from build123d import *

# Parameters (mm, degrees)
ESBO_O6_R                 = 10.25
ESBO_O6_R_2               = 8.55
FURO_ROSCADO_DE_M61_D     = 5
FURO_ROSCADO_DE_M61_DEPTH = 15
FURO_ROSCADO_DE_M61_TIP   = 1.502151548


with BuildPart() as part:
    # Varredura1: sweep along a path in Esboço5
    with BuildLine(Plane.XY) as varredura1_path:
        Line((0, 0), (-160, 0))
        ThreePointArc((-160, 0), (-174.142135624, 5.857864376), (-180, 20))
        Line((-180, 20), (-180, 260))
    # Esboço6 → Varredura1 (sweep)
    with BuildSketch(Plane.ZY):
        Circle(ESBO_O6_R)
        Circle(ESBO_O6_R_2, mode=Mode.SUBTRACT)
    sweep(path=varredura1_path.line)

    # Furo roscado de M61
    with Locations(Plane.ZY.offset(195)):
        with Locations((0, 240), (0, 215), (0, 190), (0, 165)):
            Hole(FURO_ROSCADO_DE_M61_D / 2, depth=FURO_ROSCADO_DE_M61_DEPTH)
            with Locations((0, 0, -(FURO_ROSCADO_DE_M61_DEPTH + FURO_ROSCADO_DE_M61_TIP / 2))):  # 118° drill point
                Cone(0, FURO_ROSCADO_DE_M61_D / 2, FURO_ROSCADO_DE_M61_TIP, mode=Mode.SUBTRACT)


solid = part.part
Build history of the part. All positions in model axes, mm. A direction names the side the tool comes from. Give positions to 0.01 mm unless a question says otherwise; leave off trailing zeros. Write each loop counter-clockwise with the first axis right and the second up, starting at its lowest first coordinate (ties: lowest second). Pieces come first, ordered by that corner, then holes. Notation, with made-up numbers: (80, 74.5) - (91, 74.5) arc R12 ccw to (91, 79.5) - close; hole circle Ø1 at (13, 43). An arc over 180 degrees is marked (long way). Use one line per item in the form item = value. Start each with the question number.
1. Band-saw the part on A-A on y = 49. Write the cut outline in (x, z).
2. 3-axis set-ups, long thin cutter, end or side, ignore diameter. For faces 4 (the face through (-189.198, 240.751, -2.385)), 5 (the face through (-185.3, 260, -6.9)), 6 (the face through (-81.12, -10.006, -2.222)): which of +Z, -Z, +X, -X, +Y, -Y reach the whole face in a straight line?
3. Band-saw the part on B-B on x = -132.5. Write the cut outline in (y, z), plus the area to 3 significant figures.
4. Two-plate mould, pull along X, no slides. Class faces 1 (the face through (-81.12, 2.568, 8.155)), 2 (the face through (-190.006, 141.68, -2.222)), 3 (the face through (-188.347, 141.68, -1.853)): released by +X, released by -X, zero draft, split by the parting line, or undercut.
5. Probe line 1 (X direction, y = 97, z = -0.5); line 2 (X direction, y = 245, z = -2.75); line 3 (Y direction, x = -136.5, z = 4). List the from-to ranges inside material, lowest first. Write a range as [from, to].
6. Drop flat-ended pins along their axis: pin 1 Ø4.5 at (y, z) = (165, 0) entering from -X; pin 2 Ø3 at (y, z) = (190, 0) entering from -X; pin 3 Ø1 at (x, z) = (-104, 5) entering from -Y. Give the stop position or say it passes through.
Conclusion:
q1.outline = circle Ø20.5 at (-180, 0); hole circle Ø17.1 at (-180, 0)
q2.face_4 = -X
q2.face_5 = +Z, -Z, +X, -X, +Y
q2.face_6 = +X
q3.outline = circle Ø20.5 at (0, 0); hole circle Ø17.1 at (0, 0)
q3.area = 100 mm²
q4.face_1 = zero draft
q4.face_2 = split by the parting line
q4.face_3 = undercut
q5.line_1 = [-190.24, -188.54], [-171.46, -169.76]
q5.line_2 = [-189.87, -188.1], [-171.9, -170.13]
q5.line_3 = [-9.44, -7.56], [7.56, 9.44]
q6.pin_1 = -171.75
q6.pin_2 = -171.58
q6.pin_3 = -9.21
